Source: three-view drawing plus pictorial views. Frame: mm from the lowest corner of the part. A direction names the side the tool comes from. Give positions to 0.01 mm unless a question says otherwise; leave off trailing zeros. Loops run counter-clockwise (first coordinate to the right, second up) from the corner with the lowest first, then second, coordinate; pieces in that order, holes last.
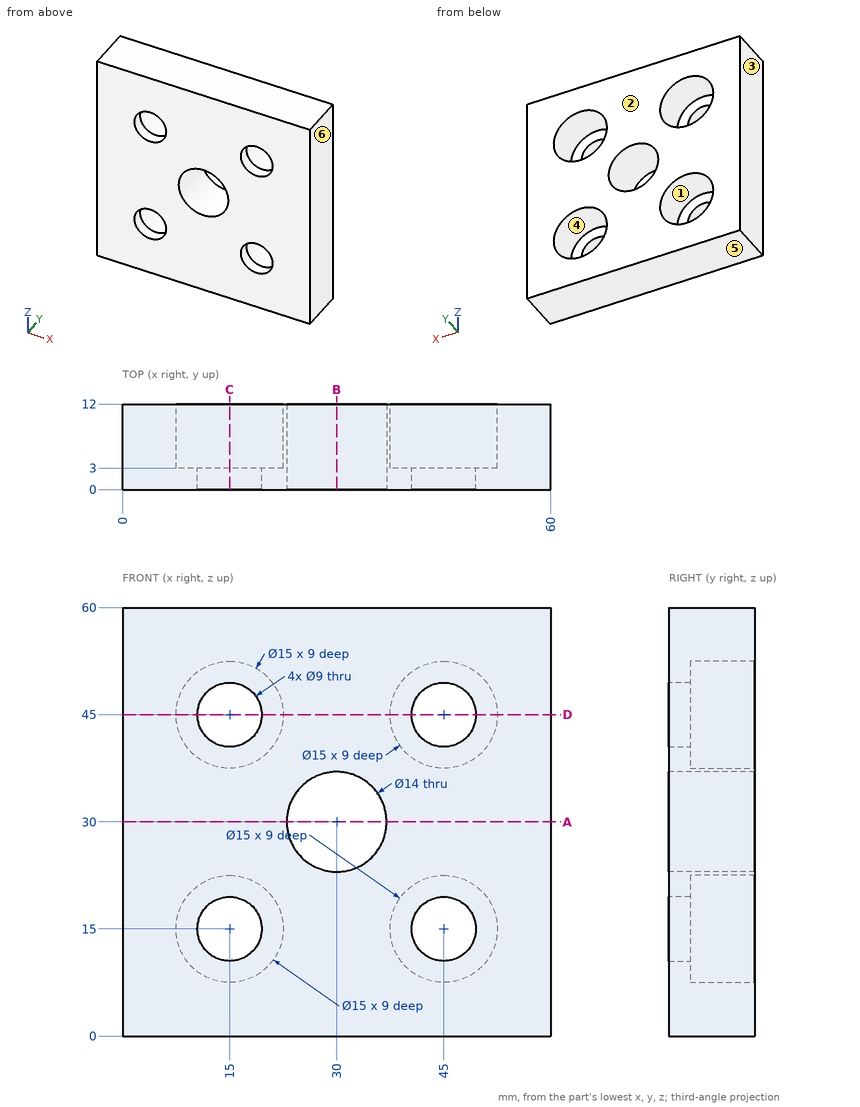
(1) Reachability of the marked faces 1 and 2 from +Z, -Z, +X, -X, +Y, -Y: full face, straight path, thin tool, end or side. Return the list, or none.
Values follow:
face 1: +Y
face 2: +Z, -Z, +X, -X, +Y
(2) Cut plane D-D (z = 45). Return the cut outline in (x, y).
Values follow:
outline: (0, 0) - (10.5, 0) - (10.5, 3) - (7.5, 3) - (7.5, 12) - (0, 12) - close; (19.5, 0) - (40.5, 0) - (40.5, 3) - (37.5, 3) - (37.5, 12) - (22.5, 12) - (22.5, 3) - (19.5, 3) - close; (49.5, 0) - (60, 0) - (60, 12) - (52.5, 12) - (52.5, 3) - (49.5, 3) - close
(3) Cut plane C-C (x = 15). Return the cut outline in (y, z), and give its area (3 significant figures).
Values follow:
outline: (0, 0) - (12, 0) - (12, 7.5) - (3, 7.5) - (3, 10.5) - (0, 10.5) - close; (0, 19.5) - (3, 19.5) - (3, 22.5) - (12, 22.5) - (12, 37.5) - (3, 37.5) - (3, 40.5) - (0, 40.5) - close; (0, 49.5) - (3, 49.5) - (3, 52.5) - (12, 52.5) - (12, 60) - (0, 60) - close
area: 396 mm2
(4) Ray query, probe 1 along X at (y, z) = (2.2, 45); probe 2 along X at (y, z) = (10, 45); probe 3 along Z at (x, y) = (50.5, 5.5). Return the intervals inside material, ascending.
Values follow:
probe 1: x = 0 to 10.5, 19.5 to 40.5, 49.5 to 60
probe 2: x = 0 to 7.5, 22.5 to 37.5, 52.5 to 60
probe 3: z = 0 to 9.9, 20.1 to 39.9, 50.1 to 60
(5) Mould query, pull axis X, two halves, no side actions, for the marked faces 3, 4, 5 and 6. Classes: +X half, -X half, draft (parallel to the pull), parting line (faces both ways), or undercut.
Values follow:
face 3: -X half
face 4: undercut
face 5: draft
face 6: +X half
(6) Pin query (flat end, axial travel): pin 1 Ø4.5 at (x, z) = (18.5, 15.5) entering from +Y. Return the tip coordinate at first contact, or that it passes through.
Values follow:
pin 1: stops at y = 3
(7) Cut plane B-B (x = 30). Return the cut outline in (y, z), and give its area (3 significant figures).
Values follow:
outline: (0, 0) - (12, 0) - (12, 23) - (0, 23) - close; (0, 37) - (12, 37) - (12, 60) - (0, 60) - close
area: 552 mm2
(8) Cut plane A-A (z = 30). Return the cut outline in (x, y), and give its area (3 significant figures).
Values follow:
outline: (0, 0) - (23, 0) - (23, 12) - (0, 12) - close; (37, 0) - (60, 0) - (60, 12) - (37, 12) - close
area: 552 mm2
